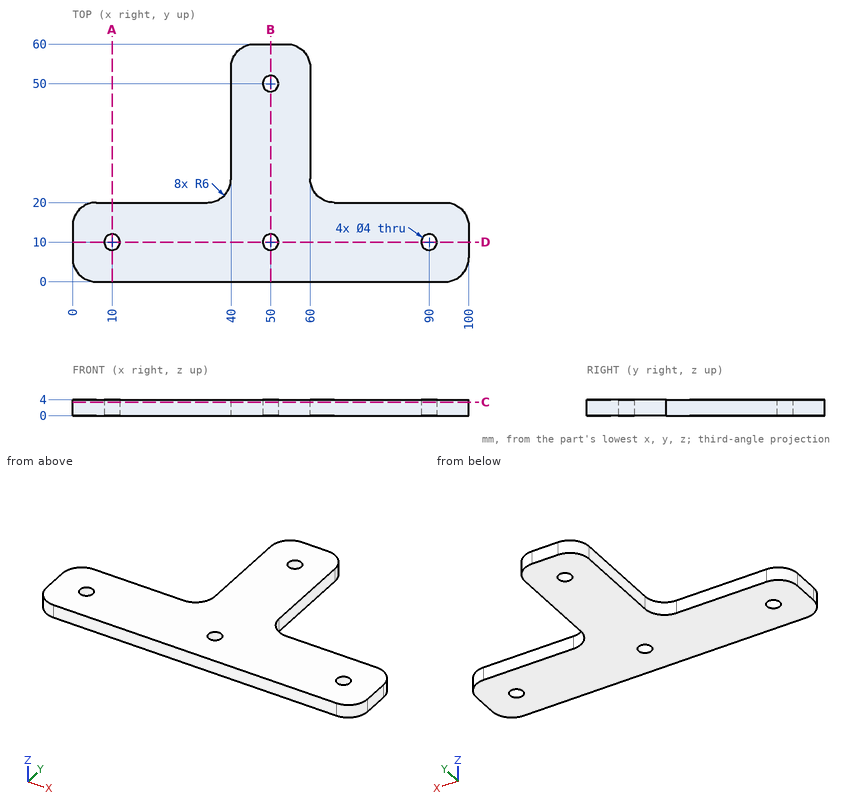
Geometry: see drawing. Coordinates: mm, zero at the bounding-box minimum. Coordinates: 2 decimals unless noted, no trailing zeros. Loops run counter-clockwise (first coordinate to the right, second up) from the corner with the lowest first, then second, coordinate; pieces in that order, holes last.
Q1. Cut plane B-B (x = 50). Output: boundary loops of the cut face in (y, z).
Q2. Cut plane C-C (z = 3.4). Output: boundary loops of the cut face in (x, y).
Q3. Material intervals for line 1 (Y direction, x = 50, z = 0.9); line 2 (Y direction, x = 49, z = 3.4); line 3 (X direction, y = 10.5, z = 3.7), sorted ascending.
Q4. Contact query for flat-ended pins moving along their axis: pin 1 (4 mm diameter, centred on x = 61, y = 46.5, fed in from -Z); pin 2 (2 mm diameter, centred on y = 41.5, z = 3, fed in from -X); pin 3 (2 mm diameter, centred on y = 44.5, z = 1, fed in from +X); pin 4 (2 mm diameter, centred on x = 76.5, z = 2, fed in from +Y). Output: stop coordinate, or through.
Q5. Cut plane D-D (y = 10). Output: boundary loops of the cut face in (x, z), then the cut area to 3 significant figures.
Q6. Cut plane A-A (x = 10). Output: boundary loops of the cut face in (y, z).
Working result:
1. outline: (0, 0) - (8, 0) - (8, 4) - (0, 4) - close; (12, 0) - (48, 0) - (48, 4) - (12, 4) - close; (52, 0) - (60, 0) - (60, 4) - (52, 4) - close
2. outline: (0, 6) arc R6 ccw to (6, 0) - (94, 0) arc R6 ccw to (100, 6) - (100, 14) arc R6 ccw to (94, 20) - (66, 20) arc R6 cw to (60, 26) - (60, 54) arc R6 ccw to (54, 60) - (46, 60) arc R6 ccw to (40, 54) - (40, 26) arc R6 cw to (34, 20) - (6, 20) arc R6 ccw to (0, 14) - close; hole circle Ø4 at (10, 10); hole circle Ø4 at (50, 10); hole circle Ø4 at (50, 50); hole circle Ø4 at (90, 10)
3. line 1: y = 0 to 8, 12 to 48, 52 to 60
3. line 2: y = 0 to 8.27, 11.73 to 48.27, 51.73 to 60
3. line 3: x = 0 to 8.06, 11.94 to 48.06, 51.94 to 88.06, 91.94 to 100
4. pin 1: stops at z = 0
4. pin 2: stops at x = 40
4. pin 3: stops at x = 60
4. pin 4: stops at y = 20
5. outline: (0, 0) - (8, 0) - (8, 4) - (0, 4) - close; (12, 0) - (48, 0) - (48, 4) - (12, 4) - close; (52, 0) - (88, 0) - (88, 4) - (52, 4) - close; (92, 0) - (100, 0) - (100, 4) - (92, 4) - close
5. area: 352 mm2
6. outline: (0, 0) - (8, 0) - (8, 4) - (0, 4) - close; (12, 0) - (20, 0) - (20, 4) - (12, 4) - close
